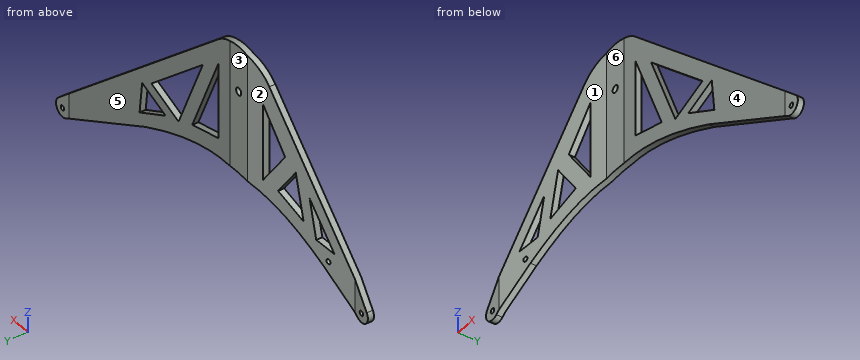
from build123d import *

# Parameters (mm, degrees)
F1_W     = 30
F1_H     = 10
F2_DEPTH = 340
F3_DEPTH = 100
F5_DEPTH = 76
F6_R     = 4
F6_R_2   = 6
F7_DEPTH = 66


with BuildPart() as f2:
    # F1 (on Top) → F2 (new body)
    with BuildSketch(Plane.XY):
        Polygon((0, 0), (-20, 0), (-20, -10), (0, -10), (20, -10), (20, 0), align=None)
        Polygon((-20, -10), (-20, 0), (-223.64854, -33), (-223.64854, -43), align=None)
        with Locations((-238.64854, -38)):
            Rectangle(F1_W, F1_H)
        Polygon((442.00493, -33), (20, 0), (20, -10), (442.00493, -43), align=None)
        with Locations((457.00493, -38)):
            Rectangle(F1_W, F1_H)
    extrude(amount=-F2_DEPTH)

    # F1 (on Top) → F3 (join)
    with BuildSketch(Plane.XY):
        Polygon((0, 0), (-20, 0), (-20, -10), (0, -10), (20, -10), (20, 0), align=None)
        Polygon((-20, -10), (-20, 0), (-223.64854, -33), (-223.64854, -43), align=None)
        with Locations((-238.64854, -38)):
            Rectangle(F1_W, F1_H)
        Polygon((442.00493, -33), (20, 0), (20, -10), (442.00493, -43), align=None)
        with Locations((457.00493, -38)):
            Rectangle(F1_W, F1_H)
    extrude(amount=F3_DEPTH)

    # F4 (on Front) → F5 (intersect, symmetric)
    with BuildSketch(Plane.XZ):
        with BuildLine():
            ThreePointArc((-250.9718022583, -230.0965111685), (-249.006915225, -249.4976876834), (-229.5356153331, -250.563010045))
            ThreePointArc((-229.5356153331, -250.563010045), (-225.2006047987, -245.2933166844), (-223.6485386505, -238.6485386505))
            ThreePointArc((-223.6485386505, -238.6485386505), (-234.1679669301, -224.3333552056), (-250.9718022583, -230.0965111685))
        make_face()
        with BuildLine():
            add(Edge.make_bspline(
                [(-229.5356153331, -250.563010045), (-208.7207010553, -234.6424785008), (-187.0701685552, -217.0301430269), (-164.0481391717, -200.4741451059)],
                knots=[0, 0, 0, 0, 0.1373195068, 0.1373195068, 0.1373195068, 0.1373195068], degree=3))
            Line((-229.5356153331, -250.563010045), (-164.0481391717, -200.4741451059))
        make_face()
        with BuildLine():
            ThreePointArc((-223.6485386505, -238.6485386505), (-225.2006047987, -245.2933166844), (-229.5356153331, -250.563010045))
            add(Edge.make_bspline(
                [(-229.5356153331, -250.563010045), (-208.7207010553, -234.6424785008), (-187.0701685552, -217.0301430269), (-164.0481391717, -200.4741451059)],
                knots=[0, 0, 0, 0, 0.1373195068, 0.1373195068, 0.1373195068, 0.1373195068], degree=3))
            Line((-164.0481391717, -200.4741451059), (0, -75))
            ThreePointArc((0, -75), (-66.4530293795, -34.7706037666), (-61.6163187638, 42.7601363655))
            Line((-61.6163187638, 42.7601363655), (-250.9718022583, -230.0965111685))
            ThreePointArc((-250.9718022583, -230.0965111685), (-234.1679669301, -224.3333552056), (-223.6485386505, -238.6485386505))
        make_face()
        with BuildLine():
            Line((0, -75), (-164.0481391717, -200.4741451059))
            add(Edge.make_bspline(
                [(-164.0481391717, -200.4741451059), (-116.7152354778, -166.4352929221), (-4.1014041633, -103.751655246), (155.4809175381, -168.4276528716), (240.7432263876, -213.1721002441)],
                knots=[0.1373195068, 0.1373195068, 0.1373195068, 0.1373195068, 0.4196460942, 0.7357326781, 0.7357326781, 0.7357326781, 0.7357326781], degree=3))
            Line((240.7432263876, -213.1721002441), (0, -75))
        make_face()
        with BuildLine():
            ThreePointArc((49.3759786376, 56.4536334843), (-9.1833788682, 74.4356470555), (-61.6163187638, 42.7601363655))
            ThreePointArc((-61.6163187638, 42.7601363655), (-66.4530293795, -34.7706037666), (0, -75))
            ThreePointArc((0, -75), (53.033008589, -53.033008589), (75, 0))
            ThreePointArc((75, 0), (68.2942105812, 30.9983999763), (49.3759786376, 56.4536334843))
        make_face()
        with BuildLine():
            ThreePointArc((75, 0), (53.033008589, -53.033008589), (0, -75))
            Line((0, -75), (240.7432263876, -213.1721002441))
            add(Edge.make_bspline(
                [(240.7432263876, -213.1721002441), (312.0276249141, -250.5811390256), (383.9898125383, -295.3870059685), (449.5382273905, -333.0078449167)],
                knots=[0.7357326781, 0.7357326781, 0.7357326781, 0.7357326781, 1, 1, 1, 1], degree=3))
            ThreePointArc((449.5382273905, -333.0078449167), (444.7952538382, -311.2848606652), (466.8801220688, -308.7075678715))
            Line((466.8801220688, -308.7075678715), (49.3759786376, 56.4536334843))
            ThreePointArc((49.3759786376, 56.4536334843), (68.2942105812, 30.9983999763), (75, 0))
        make_face()
        with BuildLine():
            add(Edge.make_bspline(
                [(240.7432263876, -213.1721002441), (312.0276249141, -250.5811390256), (383.9898125383, -295.3870059685), (449.5382273905, -333.0078449167)],
                knots=[0.7357326781, 0.7357326781, 0.7357326781, 0.7357326781, 1, 1, 1, 1], degree=3))
            Line((240.7432263876, -213.1721002441), (449.5382273905, -333.0078449167))
        make_face()
        with BuildLine():
            ThreePointArc((466.8801220688, -308.7075678715), (444.7952538382, -311.2848606652), (449.5382273905, -333.0078449167))
            ThreePointArc((449.5382273905, -333.0078449167), (464.521558007, -332.979057912), (472.0049255088, -319.9982938402))
            ThreePointArc((472.0049255088, -319.9982938402), (470.6637678536, -313.7986143485), (466.8801220688, -308.7075678715))
        make_face()
    extrude(amount=F5_DEPTH, both=True, mode=Mode.INTERSECT)

    # F6 (on face) → F7 (cut, symmetric)
    with BuildSketch(Plane.XZ.offset(10)):
        Polygon((-50, -118.8666767037), (-50, 6.8798678522), (-91.5673471808, -58.5868135927), align=None)
        Polygon((-126.4676634488, -146.9804479722), (-78.2616292159, -121.9207695), (-111.7079214913, -73.417844568), align=None)
        Polygon((-150.4108945671, -164.6469025725), (-137.8857839916, -102.2217094685), (-184.8640607304, -169.9162639715), align=None)
        Polygon((50, 16.0521292518), (50, -109.3419641256), (118.974648416, -131.2328726053), align=None)
        Polygon((225.9725652657, -131.215947327), (91.4881845235, -13.5920175816), (154.9125586599, -149.0252423531), align=None)
        Polygon((250.1992884028, -145.7627206944), (188.8613105429, -161.1354485647), (256.9922346805, -199.3553946004), align=None)
        with Locations((-238.6485386505, -238.6485386505)):
            Circle(F6_R)
        with Locations((457.0049255088, -319.9982938402)):
            Circle(F6_R)
        Circle(F6_R_2)
        with Locations((-173.5450253277, -188.5422087565)):
            Circle(F6_R)
    extrude(amount=F7_DEPTH, both=True, mode=Mode.SUBTRACT)


solid = f2.part
Can you work these out from the model? Positions are in its coordinate system, mm. Face numbers are marked on the shaded views. A direction names the side the tool comes from. Give positions to 0.01 mm unless a question says otherwise; leave off trailing zeros. Loops run counter-clockwise (first coordinate to the right, second up) from the corner with the lowest first, then second, coordinate; pieces in that order, holes last. Notation, with made-up numbers: (4, 39) -> (13, 39) arc R5 ccw to (13, 47) -> close; hole circle Ø4 at (84, 47). An arc over 180 degrees is marked (long way). Return JSON: item names as keys, results as strings.
Q1. We'd pull the mould along X, two halves only. Please class the marked faces 3, 4, 5 and 6: released by +X, released by -X, zero draft, split by the parting line, or undercut.
Checks:
{"face 3": "zero draft", "face 4": "undercut", "face 5": "released by +X", "face 6": "undercut"}
Q2. I want a section at A-A, the plane x = 313. List the corners of the cut face in (y, z) for me, then the cut area to 3 significant figures.
Checks:
{"outline": "(-32.91, -254.64) -> (-22.91, -254.64) -> (-22.91, -174.12) -> (-32.91, -174.12) -> close", "area": "805 mm2"}
Q3. I need wall thicknesses on probe 1 along X at (y, z) = (-17, -39); probe 2 along X at (y, z) = (-39.5, -230); probe 3 along Y at (x, z) = (38.5, 38.5). Which ranges of each line are inside material? Lowest first, please.
Checks:
{"probe 1": "x = -118.36 to -79.13, 120.54 to 158.51", "probe 2": "x = -250.9 to -202.65", "probe 3": "y = -11.45 to -1.45"}
Q4. For pin 1 Ø13 at (x, z) = (-238.65, -238.65) entering from +Y; pin 2 Ø13 at (x, z) = (-173.55, -188.54) entering from -Y; pin 3 Ø5 at (y, z) = (-7.5, -69) entering from -X; pin 4 Ø5 at (x, z) = (457, -320) entering from -Y, each with a flat end and sliding along its axis, tell me the tip position at first contact or that it passes through.
Checks:
{"pin 1": "stops at y = -33", "pin 2": "stops at y = -35.94", "pin 3": "stops at x = -50", "pin 4": "passes through"}
Q5. On a 3-axis mill with a long thin cutter (end or side, diameter ignored), from which of +Z, -Z, +X, -X, +Y, -Y can I reach the whole of each face in a straight line? I mean the marked faces 1 and 2. Say none if no direction works.
Checks:
{"face 1": "+Z, -Z, -Y", "face 2": "+Z, -Z, -X, +Y"}
